Could you check a few things on this drawing? It's one solid part, dimensions in mm from its lowest x, y, z. Give positions to 0.01 mm unless a question says otherwise; leave off trailing zeros. Write each loop counter-clockwise with the first axis right and the second up, starting at its lowest first coordinate (ties: lowest second). Pieces come first, ordered by that corner, then holes.
1. Suppose I cut it at B-B (y = 5). Please give me the cut outline in (x, z).
2. If I drill on probe 1 along X at (y, z) = (5, 0.5); probe 2 along X at (y, z) = (33.37, 0.8); probe 3 along Y at (x, z) = (13.75, 1.5), over which ranges is the centre line in solid material (lowest first)?
3. Suppose I cut it at A-A (x = 13.75). Please give me the cut outline in (y, z).
4. Suppose I cut it at C-C (x = 38.95). Please give me the cut outline in (y, z), and give its area (3 significant figures).
5. I'm going to push a flat-ended pin straight in: pin 1 (2.5 mm diameter, centred on x = 18.95, y = 5, fed in from +Z). Where does the tip first touch, or does it pass through?
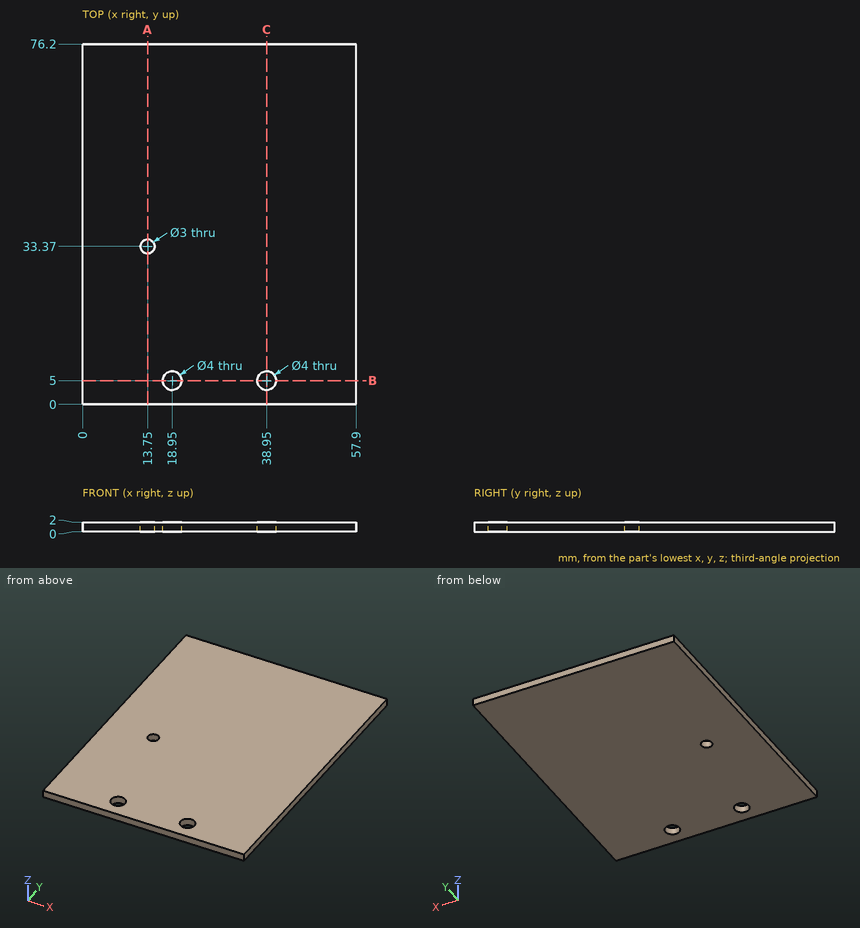
Checks:
1. outline: (0, 0) - (16.95, 0) - (16.95, 2) - (0, 2) - close; (20.95, 0) - (36.95, 0) - (36.95, 2) - (20.95, 2) - close; (40.95, 0) - (57.9, 0) - (57.9, 2) - (40.95, 2) - close
2. probe 1: x = 0 to 16.95, 20.95 to 36.95, 40.95 to 57.9
2. probe 2: x = 0 to 12.25, 15.25 to 57.9
2. probe 3: y = 0 to 31.87, 34.87 to 76.2
3. outline: (0, 0) - (31.87, 0) - (31.87, 2) - (0, 2) - close; (34.87, 0) - (76.2, 0) - (76.2, 2) - (34.87, 2) - close
4. outline: (0, 0) - (3, 0) - (3, 2) - (0, 2) - close; (7, 0) - (76.2, 0) - (76.2, 2) - (7, 2) - close
4. area: 144 mm2
5. pin 1: passes through
